Could you check a few things on this model? Use its own coordinates, in mm. A direction names the side the tool comes from. Coordinates: 2 decimals unless noted, no trailing zeros. Order: outer loops, then holes, each group sorted by start corner. A loop starts at its lowest first (then second) coordinate and runs counter-clockwise, first axis right, second up. Notation, with made-up numbers: M 85,84 L 104,84 A23 cw 104,100 Z; hole C -38.5,-36 d9. An arc over 180 degrees is marked long. Write item = value, one per line. Start each with the question number.
from build123d import *

# Parameters (mm, degrees)
F0_W     = 16.5432430804
F0_H     = 5.2285930142
F0_H_2   = 5.2797589451
F0_H_3   = 15.5384643003
F1_DEPTH = 25.4


with BuildPart() as f1:
    # F0 (on Front) → F1 (new body)
    with BuildSketch(Plane.XZ):
        Polygon((-29.214669019, 11.400138028), (-29.214669019, -11.400138028), (29.214669019, -11.400138028), (29.214669019, 11.400138028), (13.6762047186, 11.400138028), align=None)
        with BuildLine():
            add(Edge.make_bspline(
                [(-29.214669019, 11.400138028), (-10.5295465785, 20.2617670077), (8.155575862, 29.1233959875), (26.8406983024, 37.9850249672)],
                knots=[0, 0, 0, 0, 62.0399904828, 62.0399904828, 62.0399904828, 62.0399904828], degree=3))
            Line((-29.214669019, 11.400138028), (13.6762047186, 11.400138028))
            Line((13.6762047186, 11.400138028), (13.6762047186, 16.7585816234))
            ThreePointArc((13.6762047186, 16.7585816234), (17.2345044889, 29.2472343565), (26.8406983024, 37.9850249672))
        make_face()
        with BuildLine():
            Line((13.6762047186, 11.400138028), (29.214669019, 11.400138028))
            Line((29.214669019, 11.400138028), (29.214669019, 16.7585816234))
            ThreePointArc((29.214669019, 16.7585816234), (31.9669047322, 22.8678129764), (38.3662581444, 24.8542129993))
            Line((38.3662581444, 24.8542129993), (42.9420471191, 24.8542129993))
            Line((42.9420471191, 24.8542129993), (42.9420471191, 40.3926772997))
            Line((42.9420471191, 40.3926772997), (39.0692595726, 40.3926772997))
            ThreePointArc((39.0692595726, 40.3926772997), (33.2055864152, 40.0845606606), (27.5977154023, 38.3440488212))
            add(Edge.make_bspline(
                [(26.8406983024, 37.9850249672), (27.0930373357, 38.1046995852), (27.345376369, 38.2243742032), (27.5977154023, 38.3440488212)],
                knots=[62.0399904828, 62.0399904828, 62.0399904828, 62.0399904828, 62.877828783, 62.877828783, 62.877828783, 62.877828783], degree=3))
            ThreePointArc((26.8406983024, 37.9850249672), (17.2345044889, 29.2472343565), (13.6762047186, 16.7585816234))
            Line((13.6762047186, 16.7585816234), (13.6762047186, 11.400138028))
        make_face()
        with BuildLine():
            ThreePointArc((27.5977154023, 38.3440488212), (27.217619876, 38.1678831015), (26.8406983024, 37.9850249672))
            add(Edge.make_bspline(
                [(26.8406983024, 37.9850249672), (27.0930373357, 38.1046995852), (27.345376369, 38.2243742032), (27.5977154023, 38.3440488212)],
                knots=[62.0399904828, 62.0399904828, 62.0399904828, 62.0399904828, 62.877828783, 62.877828783, 62.877828783, 62.877828783], degree=3))
        make_face()
        with BuildLine():
            add(Edge.make_bspline(
                [(27.5977154023, 38.3440488212), (32.7124926413, 40.7697893188), (37.8272698802, 43.1955298163), (42.9420471191, 45.6212703139)],
                knots=[62.877828783, 62.877828783, 62.877828783, 62.877828783, 79.8603630017, 79.8603630017, 79.8603630017, 79.8603630017], degree=3))
            ThreePointArc((27.5977154023, 38.3440488212), (33.2055864152, 40.0845606606), (39.0692595726, 40.3926772997))
            Line((39.0692595726, 40.3926772997), (42.9420471191, 40.3926772997))
            Line((42.9420471191, 40.3926772997), (42.9420471191, 45.6212703139))
        make_face()
        with Locations((51.2136686593, 43.0069738068)):
            Rectangle(F0_W, F0_H)
        with Locations((51.2136686593, 22.2143335268)):
            Rectangle(F0_W, F0_H_2)
        with Locations((51.2136686593, 32.6234451495)):
            Rectangle(F0_W, F0_H_3)
        Polygon((76.0285332799, 45.6212703139), (59.4852901995, 45.6212703139), (59.4852901995, 40.3926772997), (59.4852901995, 24.8542129993), (59.4852901995, 19.5744540542), (76.0285332799, 19.5744540542), align=None)
    extrude(amount=F1_DEPTH)


solid = f1.part
(1) For faces 4 (the cylindrical face through (31.89, -12.52, 22.8)), 5 (the flat face through (23, 0, 18)), 6 (the flat face through (29.215, -13, 2)), which set-ups out of +Z, -Z, +X, -X, +Y, -Y let a thin tool reach every point of the face, with its end or its side?
(2) Please list where these lines run through material, in increasing order: probe 1 along Z at (x, y) = (56, -2.75); probe 2 along X at (y, z) = (-13.5, -5.5); probe 3 along X at (y, z) = (-14.5, 15). Write a range as from..to.
(3) Imagine slicing it at A-A on z = 2.5. List the corners of the cut face in (x, y) for me, plus the area to 3 significant figures.
(4) Thinking about a two-plate mould opening in X: for faces 1 (the flat face through (41, -13, 24.854)), 2 (the flat face through (-29.215, -13, 0)), 3 (the flat face through (0, -13, -11.4)), which applies, released by +X, released by -X, zero draft, split by the parting line, or undercut?
(5) Will these pins go through, and if not, where does the flat tip stop? P1, Ø1.6, axis at y = -7.5, z = 21, coming from the -X side; P2, Ø8, axis at x = 61.5, y = -13.5, coming from the -Z side; P3, Ø2, axis at x = 26, y = -9.5, coming from the +Z side.
Response:
q1.face_4 = -Z, +Y, -Y
q1.face_5 = +Z, -Z, +X, -X, +Y
q1.face_6 = -Z, +X, +Y, -Y
q2.probe_1 = 19.57..45.62
q2.probe_2 = -29.21..29.21
q2.probe_3 = -21.62..29.21
q3.outline = M -29.21,-25.4 L 29.21,-25.4 L 29.21,0 L -29.21,0 Z
q3.area = 1,480 mm2
q4.face_1 = undercut
q4.face_2 = released by -X
q4.face_3 = zero draft
q5.P1 = -10.66
q5.P2 = 19.57
q5.P3 = 38.06
